from build123d import *

# Parameters (mm, degrees)
SKETCH_1_R          = 13
EXTRUDE_1_DEPTH     = 7
SKETCH_2_R          = 7.1
CUT_EXTRUDE_1_DEPTH = 4
SKETCH_3_R          = 2.5
EXTRUDE_2_DEPTH     = 20
HOLE_WIZARD_M31_D   = 3.4


with BuildPart() as part:
    # Эскиз1 → Бобышка-Вытянуть1 (new body)
    with BuildSketch(Plane.XY):
        Circle(SKETCH_1_R)
    extrude(amount=EXTRUDE_1_DEPTH)

    # Эскиз2 → Вырез-Вытянуть1 (cut)
    with BuildSketch(Plane.XY.offset(7)):
        Circle(SKETCH_2_R)
    extrude(amount=-CUT_EXTRUDE_1_DEPTH, mode=Mode.SUBTRACT)

    # Эскиз3 → Бобышка-Вытянуть2 (add)
    with BuildSketch(Plane(origin=(0, 0, 0), x_dir=(-1, 0, 0), z_dir=(0, 0, -1))):
        with Locations(Location((0, 0, 0), (0, 0, 180))):
            Circle(SKETCH_3_R)
    extrude(amount=EXTRUDE_2_DEPTH)

    # Отверстие с зазором M31 (through all)
    with Locations(Plane(origin=(0, 0, 0), x_dir=(-1, 0, 0), z_dir=(0, 0, -1))):
        with Locations((0, 10), (-10, 0), (0, -10), (10, 0)):
            Hole(HOLE_WIZARD_M31_D / 2)


solid = part.part
Geometry check sheet. Reference: the model listing, model coordinates, mm. A direction names the side the tool comes from. Round coordinates to 2 decimals unless told otherwise and drop trailing zeros. Loops run counter-clockwise (first coordinate to the right, second up) from the corner with the lowest first, then second, coordinate; pieces in that order, holes last. Notation, with made-up numbers: (84, 35) - (89, 35) arc R24 ccw to (89, 61) - close; hole circle Ø7 at (81, 10). An arc over 180 degrees is marked (long way). Answer as CSV lines item,"result".
(1) Depth check by flat-ended pin: pin 1 Ø6 at (x, z) = (5, 1.5) entering from -Y; pin 2 Ø4 at (x, z) = (4, -9) entering from +Y; pin 3 Ø1.5 at (x, y) = (4, 5) entering from -Z. Enter the tip coordinate at first touch or a pass-through.
Output values:
pin 1,"stops at y = -12.85"
pin 2,"stops at y = 1.5"
pin 3,"stops at z = 0"
(2) Cross-section at D-D, the plane z = 0.5. Enter the section's corners in (x, y).
Output values:
outline,"circle Ø26 at (0, 0); hole circle Ø3.4 at (-10, 0); hole circle Ø3.4 at (0, -10); hole circle Ø3.4 at (0, 10); hole circle Ø3.4 at (10, 0)"
(3) Cross-section at B-B, the plane y = 0. Enter the section's corners in (x, z), and give its area (3 significant figures).
Output values:
outline,"(-13, 0) - (-11.7, 0) - (-11.7, 7) - (-13, 7) - close; (-8.3, 0) - (-2.5, 0) - (-2.5, -20) - (2.5, -20) - (2.5, 0) - (8.3, 0) - (8.3, 7) - (7.1, 7) - (7.1, 3) - (-7.1, 3) - (-7.1, 7) - (-8.3, 7) - close; (11.7, 0) - (13, 0) - (13, 7) - (11.7, 7) - close"
area,"178 mm²"
(4) Material ranges on line 1 along Y through (x, z) = (0, 4.5); line 2 along Z through (x, y) = (10.5, -3.25); line 3 along Z through (x, y) = (4, -2.25), recorded low to high.
Output values:
line 1,"y = -13 to -11.7, -8.3 to -7.1, 7.1 to 8.3, 11.7 to 13"
line 2,"z = 0 to 7"
line 3,"z = 0 to 3"
(5) Release check for a two-part mould opening along Y. For faces 4 (the face through (3, 0, 0)), 5 (the face through (-10.316, -7.91, 3.451)), 6 (the face through (-0.92, 7.04, 5.03)) record: released by +Y, released by -Y, zero draft, split by the parting line, or undercut.
Output values:
face 4,"zero draft"
face 5,"split by the parting line"
face 6,"undercut"
(6) Cross-section at A-A, the plane z = 5. Enter the section's corners in (x, y), and give its area (3 significant figures).
Output values:
outline,"circle Ø26 at (0, 0); hole circle Ø3.4 at (-10, 0); hole circle Ø14.2 at (0, 0); hole circle Ø3.4 at (0, -10); hole circle Ø3.4 at (0, 10); hole circle Ø3.4 at (10, 0)"
area,"336 mm²"
(7) Cross-section at C-C, the plane x = -1. Enter the section's corners in (y, z).
Output values:
outline,"(-12.96, 0) - (-11.37, 0) - (-11.37, 7) - (-12.96, 7) - close; (-8.63, 0) - (-2.29, 0) - (-2.29, -20) - (2.29, -20) - (2.29, 0) - (8.63, 0) - (8.63, 7) - (7.03, 7) - (7.03, 3) - (-7.03, 3) - (-7.03, 7) - (-8.63, 7) - close; (11.37, 0) - (12.96, 0) - (12.96, 7) - (11.37, 7) - close"
(8) Set-up check for faces 1 (the face through (0, 0, -20)), 2 (the face through (-2.5, -0.1, -9.9)), 3 (the face through (0, 0, 3)): record each of +Z, -Z, +X, -X, +Y, -Y from which the full face is reachable in a straight line by a thin tool's end or side.
Output values:
face 1,"-Z, +X, -X, +Y, -Y"
face 2,"-Z"
face 3,"+Z"
